Model file for the job. Use its own axes, mm. Face numbers are marked on the shaded views. A direction names the side the tool comes from. Coordinates: 2 decimals unless noted, no trailing zeros. Loops run counter-clockwise (first coordinate to the right, second up) from the corner with the lowest first, then second, coordinate; pieces in that order, holes last.
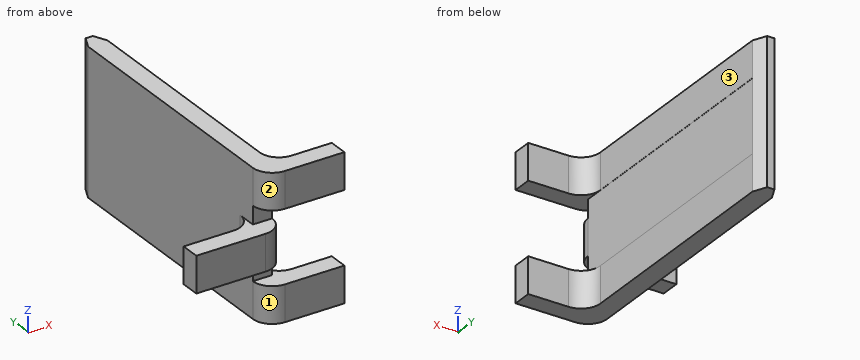
from build123d import *

# Parameters (mm, degrees)
BOSS_EXTRUDE1_DEPTH = 6.096
SKETCH2_W           = 3.048
SKETCH2_H           = 0.816265766
CUT_EXTRUDE1_DEPTH  = 10.169833116
SKETCH3_W           = 1.524
SKETCH3_H           = 0.816265766
BOSS_EXTRUDE2_DEPTH = 2.921
BOSS_EXTRUDE3_DEPTH = 1.524
SKETCH7_W           = 0.741832356
SKETCH7_H           = 3.048
CUT_EXTRUDE3_DEPTH  = 14.141059814


with BuildPart() as part:
    # Sketch1 → Boss-Extrude1 (new body)
    with BuildSketch(Plane.XY):
        with BuildLine():
            Line((0.410410125, 5.432205501), (0.1524, 5.98551))
            Line((0.1524, 5.98551), (-0.1524, 5.98551))
            Line((-0.1524, 5.98551), (-0.410410125, 5.432205501))
            Line((-0.410410125, 5.432205501), (-0.410410125, -5.169217411))
            ThreePointArc((-0.410410125, -5.169217411), (-0.169813529, -5.745269384), (0.406398179, -5.985483177))
            Line((0.406398179, -5.985483177), (2.921, -5.985483177))
            Line((2.921, -5.985483177), (2.921, -5.172683177))
            Line((2.921, -5.172683177), (1.223210125, -5.172683177))
            ThreePointArc((1.223210125, -5.172683177), (0.648473733, -4.934619569), (0.410410125, -4.359883177))
            Line((0.410410125, -4.359883177), (0.410410125, 5.432205501))
        make_face()
    extrude(amount=BOSS_EXTRUDE1_DEPTH)

    # Sketch2 → Cut-Extrude1 (cut, through all)
    with BuildSketch(Plane.ZY.offset(0.410410125)):
        with Locations((3.048, -5.577350294)):
            Rectangle(SKETCH2_W, SKETCH2_H)
    extrude(amount=-CUT_EXTRUDE1_DEPTH, mode=Mode.SUBTRACT)


with BuildPart() as body_2:
    # Sketch3 → Boss-Extrude2 (new body)
    with BuildSketch(Plane.ZY.offset(0.410410125)):
        with Locations((3.048, -5.577350294)):
            Rectangle(SKETCH3_W, SKETCH3_H)
    extrude(amount=BOSS_EXTRUDE2_DEPTH)


with BuildPart() as boss_extrude3_tool:
    # Sketch4 → Boss-Extrude3 (new body)
    with BuildSketch(Plane.XY.offset(3.81)):
        with BuildLine():
            Line((-1.223210125, -5.169217411), (-1.223210125, -5.985483177))
            Line((-1.223210125, -5.985483177), (-0.410410125, -5.985483177))
            ThreePointArc((-0.410410125, -5.985483177), (0.166164352, -5.747016402), (0.405853805, -5.170949135))
            Line((0.405853805, -5.170949135), (-0.410410125, -5.169217411))
            Line((-0.410410125, -5.169217411), (-0.410411954, -4.358141783))
            ThreePointArc((-0.410411954, -4.358141783), (-0.649083714, -4.931763137), (-1.223210125, -5.169217411))
        make_face()
    extrude(amount=-BOSS_EXTRUDE3_DEPTH)


with BuildPart() as part_1:
    add(part.part)


with BuildPart() as part_2:
    # Boss-Extrude3: joined with boss_extrude3_tool
    add(part_1.part.fuse(boss_extrude3_tool.part, body_2.part, tol=0.00001))

    # Sketch7 → Cut-Extrude3 (cut, through all)
    with BuildSketch(Plane.XZ.offset(5.169217411)):
        with Locations((0.777314357, 3.048)):
            Rectangle(SKETCH7_W, SKETCH7_H)
    extrude(amount=-CUT_EXTRUDE3_DEPTH, mode=Mode.SUBTRACT)


solid = part_2.part
Q1. Slice it at B-B (x = 2.75). List the corners of the cut face in (y, z), and give its area (3 significant figures).
Answers:
outline: (-5.99, 0) - (-5.17, 0) - (-5.17, 1.52) - (-5.99, 1.52) - close; (-5.99, 4.57) - (-5.17, 4.57) - (-5.17, 6.1) - (-5.99, 6.1) - close
area: 2.48 mm2
Q2. Flat gauge pins, fed straight in: P1, Ø0.5, axis at x = -1, y = -5.5, coming from the +Z side; P2, Ø1.7, axis at x = 1, y = -2, coming from the +Z side; P3, Ø1.7, axis at y = -0.5, z = 5.5, coming from the +X side; P4, Ø0.8, axis at x = -1, y = -5, coming from the -Z side. Where does each tip first touch, or does it go through?
Answers:
P1: stops at z = 3.81
P2: stops at z = 6.1
P3: stops at x = 0.41
P4: stops at z = 2.29
Q3. Which spindle directions (+Z, -Z, +X, -X, +Y, -Y) get a long thin tool onto all of the face, cutting with end or side? Do the marked faces 1, 2 and 3. Say none if no direction does.
Answers:
face 1: -Z, -X, -Y
face 2: +Z, -X, -Y
face 3: +Z, -Z, +X, +Y
Q4. Slice it at C-C (z = 2). List the corners of the cut face in (x, y).
Answers:
outline: (-0.41, -5.17) - (0.41, -5.17) - (0.41, 5.44) - (0.15, 5.99) - (-0.15, 5.99) - (-0.41, 5.43) - close
Q5. Drill centre lines: line 1 (Y direction, x = 2.25, z = 5.25); line 2 (X direction, y = -3.5, z = 5.75); line 3 (X direction, y = -5.5, z = 5.5). Where is each one in solid material? Low to high.
Answers:
line 1: y = -5.99 to -5.17
line 2: x = -0.41 to 0.41
line 3: x = -0.34 to 2.92
Q6. Slice it at D-D (x = -2.5). List the corners of the cut face in (y, z), and give its area (3 significant figures).
Answers:
outline: (-5.99, 2.29) - (-5.17, 2.29) - (-5.17, 3.81) - (-5.99, 3.81) - close
area: 1.24 mm2
